Input: part model. Units: mm. Frame: model coordinates. Face numbers are marked on the shaded views. A direction names the side the tool comes from. Round coordinates to 2 decimals unless told otherwise and drop trailing zeros. Order: outer loops, then holes, each group sorted by start corner. A loop starts at its lowest first (then second) coordinate and runs counter-clockwise, first axis right, second up. Notation, with made-up numbers: (-22.75, 6.25) -> (14.25, 6.25) arc R15 ccw to (14.25, 12.25) -> close; hole circle Ø10 at (-10, 34.25). An arc over 180 degrees is marked (long way). Use a Markdown table: item, result.
from build123d import *

# Parameters (mm, degrees)
F1_DEPTH  = 20
F2_R      = 1.75
F3_DEPTH  = 6
F5_DEPTH  = 3
F7_DEPTH  = 3
F8_R      = 1.75
F9_DEPTH  = 16.501
F11_DEPTH = 2.5


with BuildPart() as f1:
    # F0 (on Top) → F1 (new body)
    with BuildSketch(Plane.XY):
        Polygon((0, 10), (0, 0), (5, 0), (5, 5), (55, 5), (55, -1.5), (50, -1.5), (50, -6.5), (60, -6.5), (60, 10), align=None)
    extrude(amount=F1_DEPTH)

    # F2 (on face) → F3 (join)
    with BuildSketch(Plane(origin=(0, 0, 0), x_dir=(1, 0, 0), z_dir=(0, 0, -1))):
        Polygon((60, -39.142136), (60, -10), (35.857864, -10), (35.857864, -25), (50, -39.142136), align=None)
        with Locations((55, -34.142136)):
            Circle(F2_R, mode=Mode.SUBTRACT)
        with Locations((40.857864, -20)):
            Circle(F2_R, mode=Mode.SUBTRACT)
    extrude(amount=-F3_DEPTH)

    # F4 (on face) → F5 (cut)
    with BuildSketch(Plane.XY.offset(6)):
        Polygon((38.007864, 21.645448), (38.007864, 18.354552), (40.857864, 16.709103), (43.707864, 18.354552), (43.707864, 21.645448), (40.857864, 23.290897), align=None)
        Polygon((57.85, 32.496687), (57.85, 35.787584), (55, 37.433032), (52.15, 35.787584), (52.15, 32.496687), (55, 30.851239), align=None)
    extrude(amount=-F5_DEPTH, mode=Mode.SUBTRACT)

    # F6 (on face) → F7 (join)
    with BuildSketch(Plane.YZ.offset(60)):
        Polygon((18.082904, 6), (10, 20), (10, 6), align=None)
    extrude(amount=-F7_DEPTH)

    # F8 (on face) → F9 (cut, through all)
    with BuildSketch(Plane(origin=(0, 10, 0), x_dir=(-1, 0, 0), z_dir=(0, 1, 0))):
        with Locations((-15, 10)):
            Circle(F8_R)
    extrude(amount=-F9_DEPTH, mode=Mode.SUBTRACT)

    # F10 (on face) → F11 (cut)
    with BuildSketch(Plane(origin=(0, 10, 0), x_dir=(-1, 0, 0), z_dir=(0, 1, 0))):
        Polygon((-12.15, 8.354552), (-12.15, 11.645448), (-15, 13.290897), (-17.85, 11.645448), (-17.85, 8.354552), (-15, 6.709103), align=None)
    extrude(amount=-F11_DEPTH, mode=Mode.SUBTRACT)


solid = f1.part
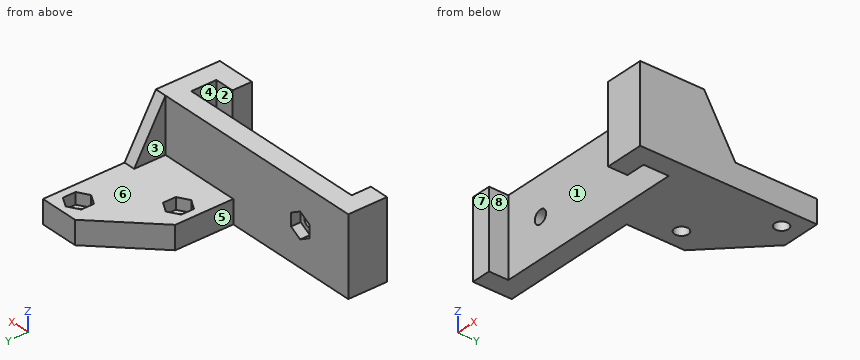
1) Pin query (flat end, axial travel): pin 1 Ø3 at (x, y) = (40.86, 20) entering from +Z; pin 2 Ø3.5 at (y, z) = (20.5, 4) entering from -X; pin 3 Ø6 at (x, z) = (42, 14.5) entering from -Y; pin 4 Ø2 at (x, z) = (27.5, 14) entering from +Y. Return the tip coordinate at first contact, or that it passes through.
Results found:
| item | result |
|---|---|
| pin 1 | passes through |
| pin 2 | stops at x = 35.86 |
| pin 3 | stops at y = 5 |
| pin 4 | stops at y = 10 |
2) Cut plane A-A on z = 4. Return loops of the section in (x, y).
Results found:
| item | result |
|---|---|
| outline | (0, 0) -> (5, 0) -> (5, 5) -> (55, 5) -> (55, -1.5) -> (50, -1.5) -> (50, -6.5) -> (60, -6.5) -> (60, 39.14) -> (50, 39.14) -> (35.86, 25) -> (35.86, 10) -> (0, 10) -> close; hole (38.01, 18.35) -> (40.86, 16.71) -> (43.71, 18.35) -> (43.71, 21.65) -> (40.86, 23.29) -> (38.01, 21.65) -> close; hole (52.15, 32.5) -> (55, 30.85) -> (57.85, 32.5) -> (57.85, 35.79) -> (55, 37.43) -> (52.15, 35.79) -> close |
3) Cut plane D-D on y = 28.5. Return loops of the section in (x, z), and give its area (3 significant figures).
Results found:
| item | result |
|---|---|
| outline | (39.36, 0) -> (60, 0) -> (60, 6) -> (39.36, 6) -> close |
| area | 124 mm² |
4) Cut plane C-C on x = 45. Return loops of the section in (y, z), and give its area (3 significant figures).
Results found:
| item | result |
|---|---|
| outline | (5, 0) -> (34.14, 0) -> (34.14, 6) -> (10, 6) -> (10, 20) -> (5, 20) -> close |
| area | 245 mm² |
5) Line query: L1, parallel to Y at x = 54, z = 9.25; L2, parallel to X at y = 1, z = 4.25; L3, parallel to X at y = 20, z = 1.8. Output: solid intervals per line, ascending. Write a range as [from, to].
Results found:
| item | result |
|---|---|
| L1 | y = [-6.5, -1.5], [5, 10] |
| L2 | x = [0, 5], [55, 60] |
| L3 | x = [35.86, 39.11], [42.61, 60] |
6) Cut plane B-B on z = 15.75. Return loops of the section in (x, y).
Results found:
| item | result |
|---|---|
| outline | (0, 0) -> (5, 0) -> (5, 5) -> (55, 5) -> (55, -1.5) -> (50, -1.5) -> (50, -6.5) -> (60, -6.5) -> (60, 12.45) -> (57, 12.45) -> (57, 10) -> (0, 10) -> close |
7) Set-up query: the marked faces 4, 5, 6, 7 and 8. Return all of +Z, -Z, +X, -X, +Y, -Y with unobstructed straight access to the full face (end or side cutting, diameter ignored); none if empty.
Results found:
| item | result |
|---|---|
| face 4 | +Z, -Z |
| face 5 | +Z, -Z, -X, +Y |
| face 6 | +Z, -X, +Y |
| face 7 | +Z, -Z, -X, -Y |
| face 8 | +Z, -Z, -Y |
8) Pull-direction query (X, two-part tool) for the marked faces 1, 2 and 3; classes: +X half, -X half, draft (parallel to the pull), parting line (faces both ways), or undercut.
Results found:
| item | result |
|---|---|
| face 1 | undercut |
| face 2 | draft |
| face 3 | -X half |
